The model under review builds one solid part; all positions refer to its coordinate system, in mm. A direction names the side the tool comes from. Coordinates: 2 decimals unless noted, no trailing zeros. Loops run counter-clockwise (first coordinate to the right, second up) from the corner with the lowest first, then second, coordinate; pieces in that order, holes last. Notation, with made-up numbers: M 55,-33.5 L 89,-33.5 A20 ccw 89,1.5 Z; hole C 31,-22 d11. An arc over 180 degrees is marked long. Return JSON: item names as keys, results as strings.
```python
from build123d import *

# Parameters (mm, degrees)
SKETCH102_W      = 5
SKETCH102_H      = 4
EXTRUDE093_DEPTH = 5
EXTRUDE064_DEPTH = 25


with BuildPart() as extrude093:
    # Sketch102 → Extrude093 (new body)
    with BuildSketch(Plane(origin=(-4, 0, 0), x_dir=(0, -1, 0), z_dir=(-1, 0, 0))):
        with Locations((-89, 2)):
            Rectangle(SKETCH102_W, SKETCH102_H)
    extrude(amount=-EXTRUDE093_DEPTH)


with BuildPart() as cut015:
    # Sketch074 → Extrude064 (new body)
    with BuildSketch(Plane.XY.offset(3)):
        Polygon((-3, 93.5), (0, 93.5), (0, 92), (-1.5, 92), (-1.5, 10.5), (0, 10.5), (0, 9), (-3, 9), align=None)
    extrude(amount=-EXTRUDE064_DEPTH)

    # Cut015: cut Extrude093
    add(extrude093.part, mode=Mode.SUBTRACT)


solid = cut015.part
```
1. To check wall thickness, follow line 1 (Y direction, x = -1.8, z = 0.75); line 2 (Y direction, x = -1.45, z = 1.25); line 3 (X direction, y = 21, z = -4.5). State the ranges of each line that lie inside material, in increasing order.
Check values:
{"line 1": "9 to 86.5, 91.5 to 93.5", "line 2": "9 to 10.5, 92 to 93.5", "line 3": "-3 to -1.5"}
2. Add section B-B on z = -4.25. Give the boundary of the cut face in (x, y), plus the area to 3 significant figures.
Check values:
{"outline": "M -3,9 L 0,9 L 0,10.5 L -1.5,10.5 L -1.5,92 L 0,92 L 0,93.5 L -3,93.5 Z", "area": "131 mm²"}
3. Insertion check: pin 1 Ø1.6 at (x, y) = (-2.5, 88) entering from +Z; pin 2 Ø7.5 at (y, z) = (38.5, -8.5) entering from +X. Each pin has a flat end and moves straight along its axis. Give the tip position at first contact, or say it passes through.
Check values:
{"pin 1": "z = 0", "pin 2": "x = -1.5"}
4. The part is to be moulded in two halves that separate along Y. For faces 4 (the face through (-2, 48, 3)), 5 (the face through (-2, 93.5, -9)), 6 (the face through (-1.5, 52, -9)), say which applies: released by +Y, released by -Y, zero draft, split by the parting line, or undercut.
Check values:
{"face 4": "zero draft", "face 5": "released by +Y", "face 6": "undercut"}
5. Add section C-C on y = 15. Give the boundary of the cut face in (x, z), plus the area to 3 significant figures.
Check values:
{"outline": "M -3,-22 L -1.5,-22 L -1.5,3 L -3,3 Z", "area": "37.5 mm²"}
6. Machinability: for faces 1 (the face through (-2, 86.5, 1)), 2 (the face through (-1, 10.5, -9)), 3 (the face through (0, 10, -9)), which of the approach directions +Z, -Z, +X, -X, +Y, -Y give a long, thin tool a straight path to every point of the face, cutting with its end or side? Answer none if there is none.
Check values:
{"face 1": "+Z, +X, -X", "face 2": "+Z, -Z, +X", "face 3": "+Z, -Z, +X, +Y, -Y"}
7. Add section A-A on z = 1.5. Give the boundary of the cut face in (x, y).
Check values:
{"outline": "M -3,9 L 0,9 L 0,10.5 L -1.5,10.5 L -1.5,86.5 L -3,86.5 Z; M -3,91.5 L -1.5,91.5 L -1.5,92 L 0,92 L 0,93.5 L -3,93.5 Z"}
